```python
from build123d import *

# Parameters (mm, degrees)
ESQUISSE1_W             = 60.96
ESQUISSE1_H             = 33.02
BOSS_EXTRU_1_DEPTH      = 1.524
ESQUISSE3_W             = 8.255
ESQUISSE3_H             = 9.9695
BOSS_EXTRU_2_DEPTH      = 3.683
BOSS_EXTRU_3_DEPTH      = 3.5052
BOSS_EXTRU_4_DEPTH      = 19.939
ENL_V_START             = -7.1882
ESQUISSE7_W             = 8.255
ESQUISSE7_H             = 0.0508
ENL_V_MAT_EXTRU_1_DEPTH = 7.1882
ESQUISSE8_W             = 3.302
ESQUISSE8_H             = 3.302
ENL_V_MAT_EXTRU_2_DEPTH = 2.032
ESQUISSE9_R             = 1.8415
ENL_V_MAT_EXTRU_3_DEPTH = 3.683
ESQUISSE10_R            = 1.5
ENL_V_MAT_EXTRU_4_DEPTH = 36.401705033


with BuildPart() as part:
    # Esquisse1 → Boss.-Extru.1 (new body)
    with BuildSketch(Plane(origin=(0, 0, 0), x_dir=(1, 0, 0), z_dir=(0, 1, 0))):
        Rectangle(ESQUISSE1_W, ESQUISSE1_H)
    extrude(amount=BOSS_EXTRU_1_DEPTH)

    # Esquisse3 → Boss.-Extru.2 (add)
    with BuildSketch(Plane(origin=(0, 1.524, 0), x_dir=(1, 0, 0), z_dir=(0, 1, 0))):
        with Locations((25.3365, -4.98475)):
            Rectangle(ESQUISSE3_W, ESQUISSE3_H)
        with Locations((25.3365, 4.98475)):
            Rectangle(ESQUISSE3_W, ESQUISSE3_H)
    extrude(amount=BOSS_EXTRU_2_DEPTH)

    # Esquisse5 → Boss.-Extru.3 (add)
    with BuildSketch(Plane(origin=(0, 5.207, 0), x_dir=(1, 0, 0), z_dir=(0, 1, 0))):
        Polygon((28.702, 0), (28.702, 9.9695), (23.586152916, 9.9695), (23.586152916, -9.9695), (28.702, -9.9695), align=None)
    extrude(amount=BOSS_EXTRU_3_DEPTH)

    # Esquisse6 → Boss.-Extru.4 (add)
    with BuildSketch(Plane.XY.offset(9.9695)):
        Polygon((23.586152916, 8.7122), (21.209, 5.207), (23.586152916, 5.207), align=None)
    extrude(amount=-BOSS_EXTRU_4_DEPTH)

    # Esquisse7 → Enlèv. mat.-Extru.1 (cut)
    with BuildSketch(Plane(origin=(0, 8.7122, 0), x_dir=(1, 0, 0), z_dir=(0, 1, 0)).offset(ENL_V_START)):
        with Locations((25.3365, 0)):
            Rectangle(ESQUISSE7_W, ESQUISSE7_H)
    extrude(amount=ENL_V_MAT_EXTRU_1_DEPTH, mode=Mode.SUBTRACT)

    # Esquisse8 → Enlèv. mat.-Extru.2 (cut)
    with BuildSketch(Plane(origin=(29.464, 0, 0), x_dir=(0, 0, -1), z_dir=(1, 0, 0))):
        with Locations((7.3025, 3.3655)):
            Rectangle(ESQUISSE8_W, ESQUISSE8_H)
        with Locations((2.6924, 3.3655)):
            Rectangle(ESQUISSE8_W, ESQUISSE8_H)
        with Locations((-7.3025, 3.3655)):
            Rectangle(ESQUISSE8_W, ESQUISSE8_H)
        with Locations((-2.6924, 3.3655)):
            Rectangle(ESQUISSE8_W, ESQUISSE8_H)
    extrude(amount=-ENL_V_MAT_EXTRU_2_DEPTH, mode=Mode.SUBTRACT)

    # Esquisse9 → Enlèv. mat.-Extru.3 (cut)
    with BuildSketch(Plane(origin=(0, 8.7122, 0), x_dir=(1, 0, 0), z_dir=(0, 1, 0))):
        with Locations(Location((26.144076458, 7.4295, 0), (0, 0, 270))):
            Circle(ESQUISSE9_R)
        with Locations(Location((26.144076458, 2.5654, 0), (0, 0, 90))):
            Circle(ESQUISSE9_R)
        with Locations(Location((26.144076458, -2.5654, 0), (0, 0, 270))):
            Circle(ESQUISSE9_R)
        with Locations(Location((26.144076458, -7.4295, 0), (0, 0, 90))):
            Circle(ESQUISSE9_R)
    extrude(amount=-ENL_V_MAT_EXTRU_3_DEPTH, mode=Mode.SUBTRACT)

    # Esquisse10 → Enlèv. mat.-Extru.4 (cut, through all)
    with BuildSketch(Plane(origin=(0, 1.524, 0), x_dir=(1, 0, 0), z_dir=(0, 1, 0))):
        with Locations(Location((-27.75, 14, 0), (0, 0, 270))):
            Circle(ESQUISSE10_R)
        with Locations(Location((27.75, 14, 0), (0, 0, 270))):
            Circle(ESQUISSE10_R)
        with Locations(Location((27.75, -14, 0), (0, 0, 270))):
            Circle(ESQUISSE10_R)
        with Locations(Location((-27.75, -14, 0), (0, 0, 270))):
            Circle(ESQUISSE10_R)
    extrude(amount=-ENL_V_MAT_EXTRU_4_DEPTH, mode=Mode.SUBTRACT)


solid = part.part
```
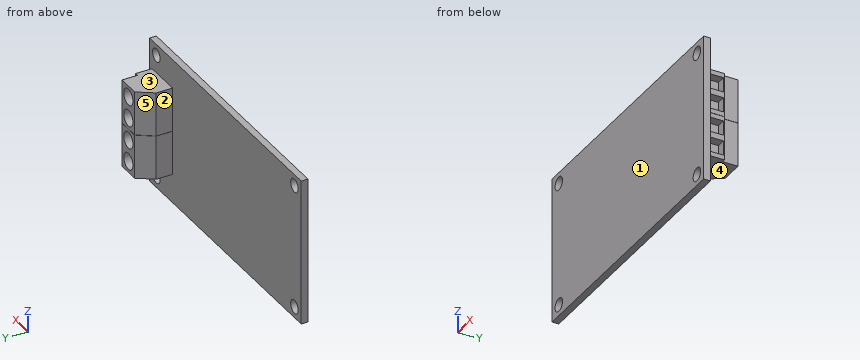
Work out the finished part from the listing and answer in its coordinate system (mm). Face numbers are marked on the shaded views. A direction names the side the tool comes from. Give positions to 0.01 mm unless a question says otherwise; leave off trailing zeros. Write each loop counter-clockwise with the first axis right and the second up, starting at its lowest first coordinate (ties: lowest second). Pieces come first, ordered by that corner, then holes. Notation, with made-up numbers: (7, -28.5) - (63, -28.5) arc R20 ccw to (63, -6.5) - close; hole circle Ø1 at (-28, 20.5). An arc over 180 degrees is marked (long way). Use one line per item in the form item = value.
1. Each of these flat-tipped pins is pushed along its axis until it touches: pin 1 Ø3.5 at (x, y) = (26.5, 5.5) entering from -Z; pin 2 Ø1.7 at (y, z) = (2.5, -6.5) entering from +X; pin 3 Ø2 at (x, z) = (26.14, 2.57) entering from +Y; pin 4 Ø3 at (x, z) = (26.5, -3) entering from +Y. Where does it stop, or does it pass through?
Filled in:
pin_1 = -9.97
pin_2 = 29.46
pin_3 = 5.03
pin_4 = 8.71
2. A cutting plane is placed at C-C (z = -14). Write down the section's boundary in (x, y).
Filled in:
outline = (-30.48, 0) - (-29.25, 0) - (-29.25, 1.52) - (-30.48, 1.52) - close; (-26.25, 0) - (26.25, 0) - (26.25, 1.52) - (-26.25, 1.52) - close; (29.25, 0) - (30.48, 0) - (30.48, 1.52) - (29.25, 1.52) - close
3. For the marked faces 1 and 2, determine the directions among +Z, -Z, +X, -X, +Y, -Y from which every point of the face is accessible in a straight line to the end or side of a thin tool.
Filled in:
face_1 = +Z, -Z, +X, -X, -Y
face_2 = +Z, -Z, -X, +Y
4. Determine the mould class of the marked faces 3, 4 and 5 for opening direction Z: released by +Z, released by -Z, zero draft, split by the parting line, or undercut.
Filled in:
face_3 = released by +Z
face_4 = released by -Z
face_5 = zero draft
5. A cutting plane is placed at B-B (x = -27.75). Write down the section's boundary in (y, z), and give its area (3 significant figures).
Filled in:
outline = (0, -16.51) - (1.52, -16.51) - (1.52, -15.5) - (0, -15.5) - close; (0, -12.5) - (1.52, -12.5) - (1.52, 12.5) - (0, 12.5) - close; (0, 15.5) - (1.52, 15.5) - (1.52, 16.51) - (0, 16.51) - close
area = 41.2 mm^2
6. A cutting plane is placed at A-A (y = 3). Write down the section's boundary in (x, z).
Filled in:
outline = (21.21, -9.97) - (29.46, -9.97) - (29.46, -8.95) - (27.43, -8.95) - (27.43, -5.65) - (29.46, -5.65) - (29.46, -4.34) - (27.43, -4.34) - (27.43, -1.04) - (29.46, -1.04) - (29.46, -0.03) - (21.21, -0.03) - close; (21.21, 0.03) - (29.46, 0.03) - (29.46, 1.04) - (27.43, 1.04) - (27.43, 4.34) - (29.46, 4.34) - (29.46, 5.65) - (27.43, 5.65) - (27.43, 8.95) - (29.46, 8.95) - (29.46, 9.97) - (21.21, 9.97) - close
7. A cutting plane is placed at D-D (y = 6.75). Write down the section's boundary in (x, z).
Filled in:
outline = (22.26, -9.97) - (28.7, -9.97) - (28.7, -0.03) - (22.26, -0.03) - close; (22.26, 0.03) - (28.7, 0.03) - (28.7, 9.97) - (22.26, 9.97) - close; hole circle Ø3.68 at (26.14, -7.43); hole circle Ø3.68 at (26.14, -2.57); hole circle Ø3.68 at (26.14, 2.57); hole circle Ø3.68 at (26.14, 7.43)
8. Consider L1, parallel to X at y = 0.55, z = -14; L2, parallel to Y at x = -11.5, z = 1.5; L3, parallel to X at y = 8, z = 7. Determine where each line is inside the solid, lowest interval first.
Filled in:
L1 = -30.48 to -29.25, -26.25 to 26.25, 29.25 to 30.48
L2 = 0 to 1.52
L3 = 23.1 to 24.35, 27.93 to 28.7
